Autodesk Inventor part; units mm, degrees
ref_plane "YZ Plane" through (0, 0, 0) normal (1, 0, 0) x (0, 1, 0)
ref_plane "XZ Plane" through (0, 0, 0) normal (0, 1, 0) x (-1, 0, 0)
ref_plane "XY Plane" through (0, 0, 0) normal (0, 0, 1) x (1, 0, 0)
sketch "スケッチ1" plane through (0, 0, 0) normal (0, 0, 1) x (1, 0, 0)
  line L0 (-70, 70) -> (70, 70)
  line L1 (70, 70) -> (70, -70)
  line L2 (70, -70) -> (-70, -70)
  line L3 (-70, -70) -> (-70, 70)
  line L4 (-62.5, 62.5) -> (62.5, 62.5) construction
  line L5 (62.5, 62.5) -> (62.5, -62.5) construction
  line L6 (62.5, -62.5) -> (-62.5, -62.5) construction
  line L7 (-62.5, -62.5) -> (-62.5, 62.5) construction
  circle A0 centre (-62.5, 62.5) radius 2.15
  line L8 (-30.5, 62.5) -> (30.5, 62.5)
  line L9 (62.5, 30.5) -> (62.5, -30.5)
  line L10 (30.5, -62.5) -> (-30.5, -62.5)
  line L11 (-62.5, -30.5) -> (-62.5, 30.5)
  arc A1 (-30.5, 62.5) -> (-62.5, 30.5) centre (-30.5, 30.5) ccw
  arc A2 (-62.5, -30.5) -> (-30.5, -62.5) centre (-30.5, -30.5) ccw
  arc A3 (30.5, -62.5) -> (62.5, -30.5) centre (30.5, -30.5) ccw
  arc A4 (62.5, 30.5) -> (30.5, 62.5) centre (30.5, 30.5) ccw
  line L12 (53.1274, 53.1274) -> (-53.1274, -53.1274) construction
  circle A5 centre (-62.5, -62.5) radius 2.15
  circle A6 centre (62.5, -62.5) radius 2.15
  circle A7 centre (62.5, 62.5) radius 2.15
  point P0 (0, 0)
  point P1 (-70, 0)
  point P2 (0, 70)
  point P3 (-62.5, 0)
  point P4 (0, 62.5)
  dimension "d0" = 140
  dimension "d1" = 125
  dimension "d3" = 4.3
  dimension "d4" = 32
  dimension "d5" = 150.267
extrude "押し出し1" add sketch "スケッチ1" along normal blind 2.2
properties part number "mesh_140" material "アルミニウム 6061"
CAD build for the part. Positions are in the model's coordinates, mm. A direction names the side the tool comes from. Coordinates: 2 decimals unless noted, no trailing zeros. Loops run counter-clockwise (first coordinate to the right, second up) from the corner with the lowest first, then second, coordinate; pieces in that order, holes last. Notation, with made-up numbers: (3, 63) - (62, 63) arc R14 cw to (62, 78) - close; hole circle Ø9 at (61.5, 55). An arc over 180 degrees is marked (long way). Use CSV: the item, a comma, the result in double quotes. Start each with the question number.
Q1. 3-axis set-ups, long thin cutter, end or side, ignore diameter. For faces 1 (the cylindrical face through (-53.37, 52.88, 1.08)), 2 (the flat face through (-63, 0, 2.2)): which of +Z, -Z, +X, -X, +Y, -Y reach the whole face in a straight line?
Q2. Cut at A-A, the plane x = -7. List the corners of the cut face in (y, z).
Q3. Cut at B-B, the plane z = 0.9. List the corners of the cut face in (x, y), then the cut area to 3 significant figures.
Q4. Two-plate mould, pull along Y, no slides. Class faces 3 (the flat face through (-63, 0, 0)), 4 (the cylindrical face through (-52.88, -53.37, 1.08)), 5 (the cylindrical face through (60.794, -61.192, 1.085)): +Y half, -Y half, draft (parallel to the pull), parting line (faces both ways), or undercut.
Q5. Probe probe 1 along Y at (x, z) = (-14, 1.25); probe 2 along X at (y, z) = (32, 1.2); probe 3 along X at (y, z) = (-42, 1.25). List the from-to ranges inside material, lowest first. Write a range as from..to.
Here are the results:
1,face 1,"+Z, -Z"
1,face 2,"+Z, +X, -X, +Y, -Y"
2,outline,"(-70, 0) - (-62.5, 0) - (-62.5, 2.2) - (-70, 2.2) - close; (62.5, 0) - (70, 0) - (70, 2.2) - (62.5, 2.2) - close"
3,outline,"(-70, -70) - (70, -70) - (70, 70) - (-70, 70) - close; hole circle Ø4.3 at (-62.5, -62.5); hole circle Ø4.3 at (-62.5, 62.5); hole (-62.5, -30.5) arc R32 ccw to (-30.5, -62.5) - (30.5, -62.5) arc R32 ccw to (62.5, -30.5) - (62.5, 30.5) arc R32 ccw to (30.5, 62.5) - (-30.5, 62.5) arc R32 ccw to (-62.5, 30.5) - close; hole circle Ø4.3 at (62.5, -62.5); hole circle Ø4.3 at (62.5, 62.5)"
3,area,"4,800 mm2"
4,face 3,"draft"
4,face 4,"undercut"
4,face 5,"undercut"
5,probe 1,"-70..-62.5, 62.5..70"
5,probe 2,"-70..-62.46, 62.46..70"
5,probe 3,"-70..-60.36, 60.36..70"
